The listing builds one solid part. Answer for the finished solid, in the listing's coordinates (mm). A direction names the side the tool comes from. Round coordinates to 2 decimals unless told otherwise and drop trailing zeros. Write each loop counter-clockwise with the first axis right and the second up, starting at its lowest first coordinate (ties: lowest second). Pieces come first, ordered by that corner, then holes. Notation, with made-up numbers: M -12.5,11.5 L 42.5,11.5 A29 ccw 42.5,46.5 Z; hole C 41.25,42.5 d10. An arc over 180 degrees is marked long. Put each result on its own line as item: value. Start each with the question number.
```python
from build123d import *

# Parameters (mm, degrees)
ESQUISSE1_W      = 30
ESQUISSE1_H      = 30
ESQUISSE1_R      = 2.25
EXTRUSION1_DEPTH = 9
ESQUISSE2_R      = 9.5
EXTRUSION2_DEPTH = 20
CHANFREIN1_SIZE  = 2
EXTRUSION3_REACH = 31
ESQUISSE3_R      = 5
CHANFREIN2_SIZE  = 0.5


with BuildPart() as part:
    # Esquisse1 → Extrusion1 (new body)
    with BuildSketch(Plane(origin=(0, 0, 0), x_dir=(1, 0, 0), z_dir=(0, 1, 0))):
        with Locations((15, 15)):
            Rectangle(ESQUISSE1_W, ESQUISSE1_H)
        with Locations((4.746951673, 25.253048327)):
            Circle(ESQUISSE1_R, mode=Mode.SUBTRACT)
        with Locations((25.253048327, 25.253048327)):
            Circle(ESQUISSE1_R, mode=Mode.SUBTRACT)
        with Locations((25.253048327, 4.746951673)):
            Circle(ESQUISSE1_R, mode=Mode.SUBTRACT)
        with Locations((4.746951673, 4.746951673)):
            Circle(ESQUISSE1_R, mode=Mode.SUBTRACT)
    extrude(amount=EXTRUSION1_DEPTH)

    # Esquisse2 → Extrusion2 (add)
    with BuildSketch(Plane(origin=(0, 9, 0), x_dir=(1, 0, 0), z_dir=(0, 1, 0))):
        with Locations((15, 15)):
            Circle(ESQUISSE2_R)
    extrude(amount=EXTRUSION2_DEPTH)

    # Chanfrein1
    chanfrein1_edges = [part.edges().sort_by_distance(p)[0] for p in [
        (0, 4.5, -30),
        (30, 4.5, -30),
        (30, 4.5, 0),
        (0, 4.5, 0),
    ]]
    chamfer(chanfrein1_edges, length=CHANFREIN1_SIZE)

    # Esquisse3 → Extrusion3 (cut, up to next)
    with BuildSketch(Plane(origin=(0, 29, 0), x_dir=(1, 0, 0), z_dir=(0, 1, 0)), mode=Mode.PRIVATE) as extrusion3_sk1:
        with Locations((15, 15)):
            Circle(ESQUISSE3_R)
    extrusion3_tool1 = extrude(extrusion3_sk1.sketch, amount=-EXTRUSION3_REACH, mode=Mode.PRIVATE) & part.part
    add(extrusion3_tool1.solids().sort_by_distance((15, 29, -15))[0], mode=Mode.SUBTRACT)

    # Chanfrein2
    chanfrein2_edges = [part.edges().sort_by_distance(p)[0] for p in [
        (5.5, 29, -15),
        (0, 9, -15),
        (15, 9, -30),
        (15, 9, 0),
        (30, 9, -15),
        (1, 9, -1),
        (29, 9, -1),
        (29, 9, -29),
        (1, 9, -29),
        (10, 0, -15),
        (10, 29, -15),
    ]]
    chamfer(chanfrein2_edges, length=CHANFREIN2_SIZE)


solid = part.part
```
Item 1: Consider line 1 along Z through (x, y) = (24.25, 5.25); line 2 along Y through (x, z) = (7.75, -24.5); line 3 along Z through (x, y) = (4.5, 6.5). Determine where each line is inside the solid, lowest interval first. Write a range as [from, to].
Item 2: Determine the mould class of faces 1 (the cylindrical face through (27.4, 4.44, -5.42)), 2 (the flat face through (28.81, 8.75, -1.16)), 3 (the flat face through (28.81, 8.75, -28.84)) for opening direction Z: released by +Z, released by -Z, zero draft, split by the parting line, or undercut.
Item 3: Section C-C (z = -4) is taken. Give the vertices of the cut face in (x, y).
Item 4: Flat-ended cylindrical pins translate along their axes: pin 1 (5 mm diameter, centred on x = 26, z = -6.5, fed in from +Y); pin 2 (3 mm diameter, centred on y = 11, z = -27, fed in from -X); pin 3 (12 mm diameter, centred on x = 5.5, y = 25, fed in from +Z); pin 4 (4 mm diameter, centred on y = 13.5, z = -12.5, fed in from +X). Find the tip coordinate at first contact, or state that the pin passes through.
Item 5: Section A-A (x = 15) is taken. Give the vertices of the cut face in (y, z).
Item 6: Which of the six approach directions +Z, -Z, +X, -X, +Y, -Y give full straight-line access (tool end or side, diameter ignored) to faces 4 (the cylindrical face through (5.51, 18.61, -15.42)), 5 (the flat face through (0, 4, -15))?
Item 7: Section B-B (z = -15) is taken. Give the vertices of the cut face in (x, y).
Item 8: Section D-D (y = 12.75) is taken. Give the vertices of the cut face in (x, z), and give its area (3 significant figures).
Output values:
1. line 1: z = [-30, -27.27], [-23.24, -6.76], [-2.73, 0]
1. line 2: y = [0, 9]
1. line 3: z = [-30, -27.49], [-23.02, -6.98], [-2.51, 0]
2. face 1: undercut
2. face 2: released by +Z
2. face 3: released by -Z
3. outline: M 0,0 L 2.62,0 L 2.62,9 L 0.5,9 L 0,8.5 Z; M 6.87,0 L 23.13,0 L 23.13,9 L 6.87,9 Z; M 27.38,0 L 30,0 L 30,8.5 L 29.5,9 L 27.38,9 Z
4. pin 1: stops at y = 9
4. pin 2: passes through
4. pin 3: stops at z = -6.17
4. pin 4: stops at x = 24.49
5. outline: M 0,-30 L 8.5,-30 L 9,-29.5 L 9,-24.5 L 28.5,-24.5 L 29,-24 L 29,-20.5 L 28.5,-20 L 0.5,-20 L 0,-20.5 Z; M 0,-9.5 L 0.5,-10 L 28.5,-10 L 29,-9.5 L 29,-6 L 28.5,-5.5 L 9,-5.5 L 9,-0.5 L 8.5,0 L 0,0 Z
6. face 4: +Y
6. face 5: +Z, -Z, -X, +Y, -Y
7. outline: M 0,0 L 9.5,0 L 10,0.5 L 10,28.5 L 9.5,29 L 6,29 L 5.5,28.5 L 5.5,9 L 0.5,9 L 0,8.5 Z; M 20,0.5 L 20.5,0 L 30,0 L 30,8.5 L 29.5,9 L 24.5,9 L 24.5,28.5 L 24,29 L 20.5,29 L 20,28.5 Z
8. outline: C 15,-15 d19; hole C 15,-15 d10
8. area: 205 mm^2
